```python
from build123d import *

# Parameters (mm, degrees)
F0_W     = 127
F0_H     = 30
F0_H_2   = 190
F1_DEPTH = 9.53
F2_DEPTH = 3.18
F4_D     = 4
F5_D     = 5
F3_W     = 127
F3_H     = 9.53
F6_DEPTH = 90.12
F8_DEPTH = 216.521
F9_D     = 12
F10_R    = 3.175


with BuildPart() as f1:
    # F0 (on Front) → F1 (new body)
    with BuildSketch(Plane.XZ):
        with Locations((0, -110)):
            Rectangle(F0_W, F0_H)
        Rectangle(F0_W, F0_H_2)
        Polygon((-63.5, 95), (63.5, 95), (63.5, 125), (35, 125), (35, 120), (-35, 120), (-35, 125), (-63.5, 125), align=None)
    extrude(amount=F1_DEPTH)

    # F0 (on Front) → F2 (join)
    with BuildSketch(Plane.XZ):
        Polygon((-63.5, 95), (63.5, 95), (63.5, 125), (35, 125), (35, 120), (-35, 120), (-35, 125), (-63.5, 125), align=None)
        with Locations((0, -110)):
            Rectangle(F0_W, F0_H)
    extrude(amount=-F2_DEPTH)

    # F4 (through all)
    with Locations(Plane.XZ.offset(9.53)):
        with Locations((-43.5, 110), (43.5, 110), (-43.5, -110), (43.5, -110)):
            Hole(F4_D / 2)

    # F5 (through all)
    with Locations(Plane(origin=(0, 0, 0), x_dir=(1, 0, 0), z_dir=(0, 1, 0))):
        with Locations((-30, 65), (30, 65)):
            Hole(F5_D / 2)

    # F3 (on face) → F6 (join)
    with BuildSketch(Plane.XZ.offset(9.53)):
        with Locations((0, 86.755)):
            Rectangle(F3_W, F3_H)
        with Locations((0, -30.235)):
            Rectangle(F3_W, F3_H)
    extrude(amount=F6_DEPTH)

    # F7 (on face) → F8 (cut, through all)
    with BuildSketch(Plane.XY.offset(91.52)):
        with BuildLine():
            Line((-30.2034766211, -69.03), (-30.9232921921, -67.03))
            ThreePointArc((-30.9232921921, -67.03), (-30.5797394754, -68.0358863166), (-30.2034766211, -69.03))
        make_face()
        with BuildLine():
            ThreePointArc((-30.2034766211, -69.03), (6.1088873707, -88.9507063689), (32.5, -57.03))
            ThreePointArc((32.5, -57.03), (-5.0617686512, -24.9265967829), (-30.9232921921, -67.03))
            Line((-30.9232921921, -67.03), (-30.2034766211, -69.03))
        make_face()
        with BuildLine():
            ThreePointArc((-54.3245395747, -69.03), (-54.9142828433, -68.0352871997), (-55.4858144033, -67.03))
            ThreePointArc((-55.4858144033, -67.03), (-61.4638072959, -52.1015012677), (-63.5, -36.15))
            Line((-63.5, -36.15), (-63.5, -99.65))
            Line((-63.5, -99.65), (2.176e-07, -99.65))
            ThreePointArc((2.176e-07, -99.65), (-20.0212042966, -96.4111100007), (-38, -87.0248464371))
            ThreePointArc((-38, -87.0248464371), (-43.5829123177, -82.3320284732), (-48.5909003827, -77.03))
            ThreePointArc((-48.5909003827, -77.03), (-51.6129532715, -73.1412564614), (-54.3245395747, -69.03))
        make_face()
        with BuildLine():
            ThreePointArc((38, -87.0248464371), (20.0212045031, -96.4111099321), (2.176e-07, -99.65))
            Line((2.176e-07, -99.65), (63.5, -99.65))
            Line((63.5, -99.65), (63.5, -36.15))
            ThreePointArc((63.5, -36.15), (59.6564002195, -57.9069279277), (48.5909003827, -77.03))
            ThreePointArc((48.5909003827, -77.03), (43.5829123177, -82.3320284732), (38, -87.0248464371))
        make_face()
        with BuildLine():
            Line((-38, -77.03), (-48.5909003827, -77.03))
            ThreePointArc((-48.5909003827, -77.03), (-43.5829123177, -82.3320284732), (-38, -87.0248464371))
            Line((-38, -87.0248464371), (-38, -77.03))
        make_face()
        with BuildLine():
            Line((38, -77.03), (38, -87.0248464371))
            ThreePointArc((38, -87.0248464371), (43.5829123177, -82.3320284732), (48.5909003827, -77.03))
            Line((48.5909003827, -77.03), (38, -77.03))
        make_face()
        with BuildLine():
            ThreePointArc((-30.2034766211, -69.03), (-30.5797394754, -68.0358863166), (-30.9232921921, -67.03))
            Line((-30.9232921921, -67.03), (-55.4858144033, -67.03))
            ThreePointArc((-55.4858144033, -67.03), (-54.9142828433, -68.0352871997), (-54.3245395747, -69.03))
            Line((-54.3245395747, -69.03), (-30.2034766211, -69.03))
        make_face()
    extrude(amount=-F8_DEPTH, mode=Mode.SUBTRACT)

    # F9 (through all)
    with Locations(Plane.XY.offset(91.52)):
        with Locations((45, -63.53)):
            Hole(F9_D / 2)

    # F10
    f10_edges = [f1.edges().sort_by_distance(p)[0] for p in [
        (-38, -77.03, 86.755),
        (-38, -77.03, -30.235),
        (38, -77.03, -30.235),
        (38, -77.03, 86.755),
        (-35, -3.175, 120),
        (35, -3.175, 120),
    ]]
    fillet(f10_edges, radius=F10_R)


solid = f1.part
```
Could you check a few things on this model? Use its own coordinates, in mm. A direction names the side the tool comes from. Round coordinates to 2 decimals unless told otherwise and drop trailing zeros. Loops run counter-clockwise (first coordinate to the right, second up) from the corner with the lowest first, then second, coordinate; pieces in that order, holes last.
Q1. I want a section at C-C (y = -74). Write out the boundary of the cut face in (x, z), and give its area (3 significant figures).
Q2. I want a section at A-A (y = -22). Write out the boundary of the cut face in (x, z), and give its area (3 significant figures).
Q3. For P1, Ø4, axis at x = -30, z = -65, coming from the -Y side; P2, Ø1.5, axis at x = -18.5, y = -24, coming from the -Z side; P3, Ø7.5, axis at x = -42.5, z = 87, coming from the +Y side; P4, Ø1.6, axis at x = -14, y = 2, coming from the +Z side, each with a flat end and sliding along its axis, tell me the tip position at first contact or that it passes through.
Q4. I want a section at B-B (z = -65). Write out the boundary of the cut face in (x, y), and give its area (3 significant figures).
Q5. Please list where these lines run through material, in increasing order: L1, parallel to Z at x = 30, y = -5.75; L2, parallel to Z at x = -8.5, y = -90; L3, parallel to Y at x = 45, z = 87.75.
Q6. On a 3-axis mill with a long thin cutter (end or side, diameter ignored), from which of +Z, -Z, +X, -X, +Y, -Y can I reach the whole of each face in a straight line? I mean faces 4 (the flat face through (-38, -84, 87)), 5 (the flat face through (0, -3, 120)), 6 (the flat face through (-1, -24, -35)), 7 (the flat face through (45, -77.03, -30)). Say none if no direction works.
Q7. I want a section at D-D (x = 21.5). Write out the boundary of the cut face in (y, z).
Q8. Thinking about a two-plate mould opening in Y: for faces 1 (the flat face through (-63.5, -8, 2)), 2 (the flat face through (-45, -77.03, 87)), 3 (the flat face through (-43, -67.03, 87)), which applies, pulls with the +Y half, pulls with the -Y half, needs draft (parallel to the pull), parting line crosses it, or undercut?
Answer below:
1. outline: (-50.99, -35) - (-27.72, -35) - (-27.72, -25.47) - (-50.99, -25.47) - close; (-50.99, 81.99) - (-27.72, 81.99) - (-27.72, 91.52) - (-50.99, 91.52) - close; (27.72, -35) - (50.99, -35) - (50.99, -25.47) - (27.72, -25.47) - close; (27.72, 81.99) - (50.99, 81.99) - (50.99, 91.52) - (27.72, 91.52) - close
1. area: 887 mm2
2. outline: (-63.5, -35) - (63.5, -35) - (63.5, -25.47) - (-63.5, -25.47) - close; (-63.5, 81.99) - (63.5, 81.99) - (63.5, 91.52) - (-63.5, 91.52) - close
2. area: 2,420 mm2
3. P1: passes through
3. P2: stops at z = -35
3. P3: stops at y = 0
3. P4: stops at z = 120
4. outline: (-63.5, -9.53) - (-32.5, -9.53) - (-32.5, 0) - (-63.5, 0) - close; (-27.5, -9.53) - (27.5, -9.53) - (27.5, 0) - (-27.5, 0) - close; (32.5, -9.53) - (63.5, -9.53) - (63.5, 0) - (32.5, 0) - close
4. area: 1,120 mm2
5. L1: z = -125 to -67.5, -62.5 to 120
5. L2: z = -35 to -25.47, 81.99 to 91.52
5. L3: y = -77.03 to -69.53, -57.53 to 0
6. face 4: +Z, -Z, -X, -Y
6. face 5: +Z, +Y, -Y
6. face 6: -Z, +X, -X, -Y
6. face 7: +Z, -Z, +X, -Y
7. outline: (-95.9, -35) - (-81.4, -35) - (-81.4, -25.47) - (-95.9, -25.47) - close; (-95.9, 81.99) - (-81.4, 81.99) - (-81.4, 91.52) - (-95.9, 91.52) - close; (-32.66, -35) - (-9.53, -35) - (-9.53, -125) - (3.18, -125) - (3.18, -95) - (0, -95) - (0, 95) - (3.18, 95) - (3.18, 120) - (-9.53, 120) - (-9.53, 91.52) - (-32.66, 91.52) - (-32.66, 81.99) - (-9.53, 81.99) - (-9.53, -25.47) - (-32.66, -25.47) - close
8. face 1: needs draft
8. face 2: pulls with the -Y half
8. face 3: undercut
